Can you work these out from the drawing? Everything is in mm from the part's minimum corner. A direction names the side the tool comes from. Give positions to 0.01 mm unless a question says otherwise; leave off trailing zeros. Write each loop counter-clockwise with the first axis right and the second up, starting at its lowest first coordinate (ties: lowest second). Pieces come first, ordered by that corner, then holes. Notation, with made-up numbers: (-32, -39.75) -> (9, -39.75) arc R28 cw to (9, -19.75) -> close; hole circle Ø2 at (3, -14.75). An arc over 180 degrees is marked (long way). Answer as CSV lines item,"result". Start each with the question number.
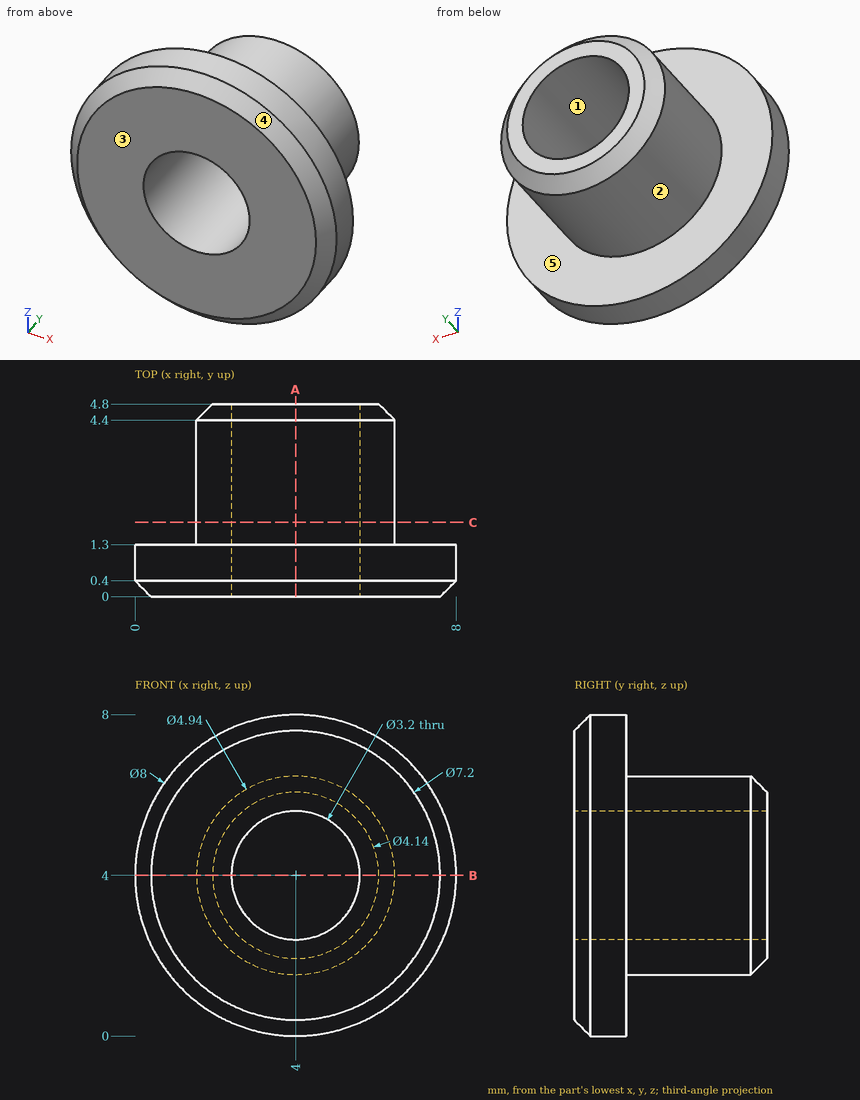
Item 1: If I drill on line 1 (Z direction, x = 4, y = 3.2); line 2 (Y direction, x = 6.5, z = 3.5); line 3 (X direction, y = 0.5, z = 3.5), over which ranges is the centre line in solid material (lowest first)? Write a range as [from, to].
Item 2: I'm going to push a flat-ended pin straight in: pin 1 (1.5 mm diameter, centred on x = 3.5, z = 6.5, fed in from +Y). Where does the tip first touch, or does it pass through?
Item 3: If we section it at B-B (z = 4): Please give me the cut outline in (x, y).
Item 4: We'd pull the mould along X, two halves only. Please class the marked faces 1, 2 and 3: released by +X, released by -X, zero draft, split by the parting line, or undercut.
Item 5: If we section it at A-A (x = 4): Please give me the cut outline in (y, z).
Item 6: If we section it at C-C (y = 1.85): Please give me the cut outline in (x, z).
Item 7: For the marked faces 4 and 5, which set-ups out of +Z, -Z, +X, -X, +Y, -Y let a thin tool reach every point of the face, with its end or its side?
Final values:
1,line 1,"[1.53, 2.4], [5.6, 6.47]"
1,line 2,"[0, 1.3]"
1,line 3,"[0.03, 2.48], [5.52, 7.97]"
2,pin 1,"y = 4.8"
3,outline,"(0, 0.4) -> (0.4, 0) -> (2.4, 0) -> (2.4, 4.8) -> (1.93, 4.8) -> (1.53, 4.4) -> (1.53, 1.3) -> (0, 1.3) -> close; (5.6, 0) -> (7.6, 0) -> (8, 0.4) -> (8, 1.3) -> (6.47, 1.3) -> (6.47, 4.4) -> (6.07, 4.8) -> (5.6, 4.8) -> close"
4,face 1,"undercut"
4,face 2,"split by the parting line"
4,face 3,"zero draft"
5,outline,"(0, 0.4) -> (0.4, 0) -> (1.3, 0) -> (1.3, 1.53) -> (4.4, 1.53) -> (4.8, 1.93) -> (4.8, 2.4) -> (0, 2.4) -> close; (0, 5.6) -> (4.8, 5.6) -> (4.8, 6.07) -> (4.4, 6.47) -> (1.3, 6.47) -> (1.3, 8) -> (0.4, 8) -> (0, 7.6) -> close"
6,outline,"circle Ø4.94 at (4, 4); hole circle Ø3.2 at (4, 4)"
7,face 4,"-Y"
7,face 5,"+Y"
